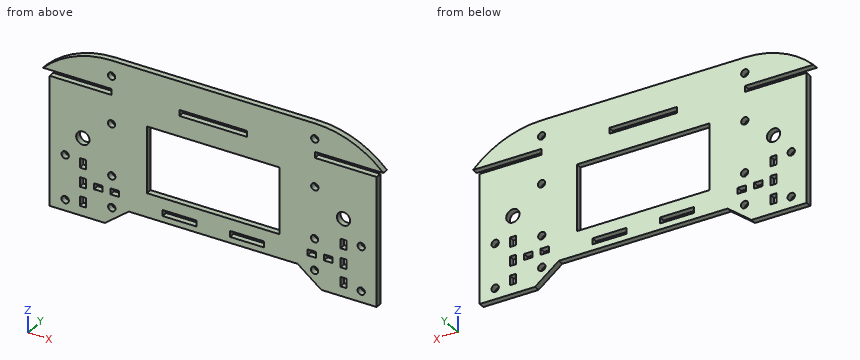
from build123d import *

# Parameters (mm, degrees)
SKETCH1_R           = 1.65
SKETCH1_R_2         = 3
SKETCH1_W           = 30.68
SKETCH1_H           = 2.7
SKETCH1_W_2         = 15.28
SKETCH1_W_3         = 2.7
SKETCH1_H_2         = 4.285714286
SKETCH1_W_4         = 3.73
SKETCH1_W_5         = 60
SKETCH1_H_3         = 30
BOSS_EXTRUDE1_DEPTH = 2.7


with BuildPart() as part:
    # Sketch1 → Boss-Extrude1 (new body)
    with BuildSketch(Plane(origin=(0, 0, 0), x_dir=(1, 0, 0), z_dir=(0, 1, 0))):
        with BuildLine():
            Line((-46, 0), (46, 0))
            ThreePointArc((46, 0), (62.780941571, 3.32568378), (77.025151087, 12.8))
            Line((77.025151087, 12.8), (46.015151087, 12.8))
            Line((46.015151087, 12.8), (46.015151087, 15.5))
            Line((46.015151087, 15.5), (73.995151087, 15.5))
            Line((73.995151087, 15.5), (73.995151087, 35.5))
            Line((73.995151087, 35.5), (73.995151087, 43.92))
            Line((73.995151087, 43.92), (73.995151087, 73.92))
            Line((73.995151087, 73.92), (68.995151087, 73.92))
            Line((68.995151087, 73.92), (48.995151087, 73.92))
            Line((48.995151087, 73.92), (38.2, 65.5))
            Line((38.2, 65.5), (-38.2, 65.5))
            Line((-38.2, 65.5), (-48.995151087, 73.92))
            Line((-48.995151087, 73.92), (-68.995151087, 73.92))
            Line((-68.995151087, 73.92), (-73.995151087, 73.92))
            Line((-73.995151087, 73.92), (-73.995151087, 15.5))
            Line((-73.995151087, 15.5), (-46.015151087, 15.5))
            Line((-46.015151087, 15.5), (-46.015151087, 12.8))
            Line((-46.015151087, 12.8), (-77.025151087, 12.8))
            ThreePointArc((-77.025151087, 12.8), (-62.780941571, 3.32568378), (-46, 0))
        make_face()
        with Locations((46, 28.5)):
            Circle(SKETCH1_R, mode=Mode.SUBTRACT)
        with Locations((46, 7)):
            Circle(SKETCH1_R, mode=Mode.SUBTRACT)
        with Locations((-46, 7)):
            Circle(SKETCH1_R, mode=Mode.SUBTRACT)
        with Locations((-46, 28.5)):
            Circle(SKETCH1_R, mode=Mode.SUBTRACT)
        with Locations((66.995151087, 68.959972417)):
            Circle(SKETCH1_R, mode=Mode.SUBTRACT)
        with Locations((66.995151087, 48.880027583)):
            Circle(SKETCH1_R, mode=Mode.SUBTRACT)
        with Locations((45.892266276, 66.076819007)):
            Circle(SKETCH1_R, mode=Mode.SUBTRACT)
        with Locations((45.892266276, 51.843125828)):
            Circle(SKETCH1_R, mode=Mode.SUBTRACT)
        with Locations((-66.995151087, 48.880027583)):
            Circle(SKETCH1_R, mode=Mode.SUBTRACT)
        with Locations((-45.892266276, 66.076819007)):
            Circle(SKETCH1_R, mode=Mode.SUBTRACT)
        with Locations((-66.995151087, 68.959972417)):
            Circle(SKETCH1_R, mode=Mode.SUBTRACT)
        with Locations((-45.892266276, 51.843125828)):
            Circle(SKETCH1_R, mode=Mode.SUBTRACT)
        with Locations((-58.995151087, 38.92)):
            Circle(SKETCH1_R_2, mode=Mode.SUBTRACT)
        with Locations((58.995151087, 38.92)):
            Circle(SKETCH1_R_2, mode=Mode.SUBTRACT)
        with Locations((0, 14.15)):
            Rectangle(SKETCH1_W, SKETCH1_H, mode=Mode.SUBTRACT)
        with Locations((-15.28, 61.45)):
            Rectangle(SKETCH1_W_2, SKETCH1_H, mode=Mode.SUBTRACT)
        with Locations((15.28, 61.45)):
            Rectangle(SKETCH1_W_2, SKETCH1_H, mode=Mode.SUBTRACT)
        with Locations((58.995151087, 58.959972417)):
            Rectangle(SKETCH1_W_3, SKETCH1_H_2, mode=Mode.SUBTRACT)
        with Locations((44.590151087, 58.927994483)):
            Rectangle(SKETCH1_W_4, SKETCH1_H, mode=Mode.SUBTRACT)
        with Locations((58.995151087, 50.388543846)):
            Rectangle(SKETCH1_W_3, SKETCH1_H_2, mode=Mode.SUBTRACT)
        with Locations((58.995151087, 67.531400989)):
            Rectangle(SKETCH1_W_3, SKETCH1_H_2, mode=Mode.SUBTRACT)
        with Locations((52.050151087, 58.94398345)):
            Rectangle(SKETCH1_W_4, SKETCH1_H, mode=Mode.SUBTRACT)
        with Locations((-52.050151087, 58.94398345)):
            Rectangle(SKETCH1_W_4, SKETCH1_H, mode=Mode.SUBTRACT)
        with Locations((-44.590151087, 58.927994483)):
            Rectangle(SKETCH1_W_4, SKETCH1_H, mode=Mode.SUBTRACT)
        with Locations((-58.995151087, 67.531400989)):
            Rectangle(SKETCH1_W_3, SKETCH1_H_2, mode=Mode.SUBTRACT)
        with Locations((-58.995151087, 58.959972417)):
            Rectangle(SKETCH1_W_3, SKETCH1_H_2, mode=Mode.SUBTRACT)
        with Locations((-58.995151087, 50.388543846)):
            Rectangle(SKETCH1_W_3, SKETCH1_H_2, mode=Mode.SUBTRACT)
        with Locations((0, 39.71)):
            Rectangle(SKETCH1_W_5, SKETCH1_H_3, mode=Mode.SUBTRACT)
    extrude(amount=BOSS_EXTRUDE1_DEPTH)


solid = part.part
Part model, mm, in its own coordinate system. Coordinates: 2 decimals unless noted, no trailing zeros. Order: outer loops, then holes, each group sorted by start corner. A loop starts at its lowest first (then second) coordinate and runs counter-clockwise, first axis right, second up. Notation, with made-up numbers: (-37, -24.5) - (-2, -24.5) arc R24 ccw to (-2, -14.5) - close; hole circle Ø4 at (-1, 45). An arc over 180 degrees is marked (long way). Use CSV: the item, a comma, the result in double quotes.
Item 1: Saw through at D-D on x = -33. Give the cut face in (y, z), and give its area (3 significant figures).
Solved:
outline,"(0, -65.5) - (2.7, -65.5) - (2.7, 0) - (0, 0) - close"
area,"177 mm²"
Item 2: Drop flat-ended pins along their axis: P1, Ø1.4, axis at y = 2, z = -41, coming from the -X side; P2, Ø1.3, axis at y = 0.5, z = -14, coming from the +X side; P3, Ø0.8, axis at x = -58.5, y = 2, coming from the +Z side; P4, Ø2, axis at x = 67, z = -48.88, coming from the -Y side. Give the stop position or say it passes through.
Solved:
P1,"stops at x = -74"
P2,"stops at x = 46.02"
P3,"stops at z = -1.7"
P4,"passes through"
Item 3: Saw through at B-B on x = -0.5. Give the cut face in (y, z).
Solved:
outline,"(0, -65.5) - (2.7, -65.5) - (2.7, -54.71) - (0, -54.71) - close; (0, -24.71) - (2.7, -24.71) - (2.7, -15.5) - (0, -15.5) - close; (0, -12.8) - (2.7, -12.8) - (2.7, 0) - (0, 0) - close"
Item 4: Saw through at C-C on z = -7. Give the cut face in (x, y).
Solved:
outline,"(-69.81, 0) - (-47.65, 0) - (-47.65, 2.7) - (-69.81, 2.7) - close; (-44.35, 0) - (44.35, 0) - (44.35, 2.7) - (-44.35, 2.7) - close; (47.65, 0) - (69.81, 0) - (69.81, 2.7) - (47.65, 2.7) - close"
Item 5: Saw through at A-A on z = -34.5. Give the cut face in (x, y), and give its area (3 significant figures).
Solved:
outline,"(-74, 0) - (-30, 0) - (-30, 2.7) - (-74, 2.7) - close; (30, 0) - (74, 0) - (74, 2.7) - (30, 2.7) - close"
area,"238 mm²"
Item 6: Probe probe 1 along Z at (x, y) = (-18, 1.35); probe 2 along Z at (x, y) = (7.5, 1.55); probe 3 along X at (y, z) = (1.1, -28.5). List the from-to ranges inside material, lowest first.
Solved:
probe 1,"z = -65.5 to -62.8, -60.1 to -54.71, -24.71 to 0"
probe 2,"z = -65.5 to -54.71, -24.71 to -15.5, -12.8 to 0"
probe 3,"x = -74 to -47.65, -44.35 to -30, 30 to 44.35, 47.65 to 74"
